Can you work these out from the model? Positions are in its coordinate system, mm. A direction names the side the tool comes from. Coordinates: 2 decimals unless noted, no trailing zeros. Loops run counter-clockwise (first coordinate to the right, second up) from the corner with the lowest first, then second, coordinate; pieces in that order, holes last.
```python
from build123d import *

# Parameters (mm, degrees)
F3_R = 7.62
F4_R = 12.7
F5_R = 5.08


with BuildPart() as f2:
    # F0 (on Front) → F2 (revolve)
    with BuildSketch(Plane.XZ):
        Polygon((0, -63.08393), (0, -66.25893), (44.45, -66.25893), (44.45, 149.64107), (19.05, 164.431536), (19.05, 187.74107), (20.699778, 187.74107), (20.699778, 189.058036), (15.875, 189.058036), (15.875, 162.606284), (41.275, 147.815819), (41.275, -63.08393), align=None)
    revolve(axis=Axis((0, 0, 62.210336), (0, 0, 1)))

    # F3
    f3_edges = [f2.edges().sort_by_distance(p)[0] for p in [
        (-44.45, 0, -66.25893),
    ]]
    fillet(f3_edges, radius=F3_R)

    # F4
    f4_edges = [f2.edges().sort_by_distance(p)[0] for p in [
        (-44.45, 0, 149.64107),
    ]]
    fillet(f4_edges, radius=F4_R)

    # F5
    f5_edges = [f2.edges().sort_by_distance(p)[0] for p in [
        (-19.05, 0, 164.431536),
    ]]
    fillet(f5_edges, radius=F5_R)


solid = f2.part
```
(1) If I drill on probe 1 along X at (y, z) = (-1, 129); probe 2 along Y at (x, z) = (0, 170) (3 decimals); probe 3 along Y at (x, z) = (0, 64) (3 decimals), over which ranges is the centre line in solid material (lowest first)?
Check values:
probe 1: x = -44.44 to -41.26, 41.26 to 44.44
probe 2: y = -19.05 to -15.875, 15.875 to 19.05
probe 3: y = -44.45 to -41.275, 41.275 to 44.45
(2) I want a section at A-A on z = 52. Write out the boundary of the cut face in (x, y) (3 decimals), then the cut area to 3 significant figures.
Check values:
outline: circle Ø88.9 at (0, 0); hole circle Ø82.55 at (0, 0)
area: 855 mm2
(3) Which directions (+Z, -Z, +X, -X, +Y, -Y) give clear straight access to the entire face, cutting with the end or side of a thin tool? Please do faces 4 (the cylindrical face through (18.17, 5.72, 177.69)), 5 (the cylindrical face through (-4.487, -20.208, 188.409)), 6 (the cylindrical face through (41.061, -17.025, 43.257)).
Check values:
face 4: none
face 5: +Z
face 6: +Z, -Z
(4) I'm going to push flat-ended pins straight in: pin 1 (6 mm diameter, centred on y = 8.5, z = 135.5, fed in from +X); pin 2 (1 mm diameter, centred on x = 7.5, y = 27.5, fed in from +Z); pin 3 (5 mm diameter, centred on x = 6, y = -3.5, fed in from +Z); pin 4 (25 mm diameter, centred on x = -5.5, y = 20.5, fed in from +Z). Where does each tip first touch, or does it pass through?
Check values:
pin 1: stops at x = 44.11
pin 2: stops at z = 159.22
pin 3: stops at z = -63.08
pin 4: stops at z = 189.06
(5) If we mould it in two halves opening along Z, with no side actions, what happens to faces 1 (the flat face through (-1, 1, -63.084)), 2 (the flat face through (1, 1, -66.259)), 3 (the cylindrical face through (-3.441, -15.497, 175.647))? For each: released by +Z, released by -Z, zero draft, split by the parting line, or undercut.
Check values:
face 1: undercut
face 2: released by -Z
face 3: zero draft
